from build123d import *

# Parameters (mm, degrees)
SKETCH1_R               = 18
SKETCH1_R_2             = 35
BOSS_EXTRUDE1_DEPTH     = 15
SKETCH1_3_R             = 35
SKETCH1_3_R_2           = 18
BOSS_EXTRUDE2_DEPTH     = 119
SKETCH1_4_R             = 18
SKETCH1_4_R_2           = 9
BOSS_EXTRUDE3_DEPTH     = 19
SKETCH1_5_W             = 56
SKETCH1_5_H             = 75
BOSS_EXTRUDE4_DEPTH     = 65
SKETCH2_R               = 14
CUT_EXTRUDE1_DEPTH      = 85.30367726
CUT_EXTRUDE1_DEPTH_BACK = 65
SKETCH3_R               = 24
SKETCH3_R_2             = 12.5
BOSS_EXTRUDE5_DEPTH     = 65
SKETCH1_6_R             = 18
CUT_EXTRUDE3_DEPTH      = 263
SKETCH3_3_R             = 12.5
CUT_EXTRUDE4_DEPTH      = 263


with BuildPart() as part:
    # Sketch1 → Boss-Extrude1 (new body)
    with BuildSketch(Plane(origin=(0, 0, 0), x_dir=(1, 0, 0), z_dir=(0, 1, 0))):
        with BuildLine():
            ThreePointArc((23.30367726, -61), (10.58036287, -81.76336426), (-13.696259751, -79.854013967))
            Line((-13.696259751, -79.854013967), (-72, -37.5))
            Line((-72, -37.5), (-72, 37.5))
            Line((-72, 37.5), (-15.87486298, 86.999686813))
            ThreePointArc((-15.87486298, 86.999686813), (9.874292088, 90.874605271), (24, 69))
            Line((24, 69), (24, 38.065732621))
            ThreePointArc((24, 38.065732621), (44.998138968, -0.409254655), (23.30367726, -38.495955971))
            Line((23.30367726, -38.495955971), (23.30367726, -61))
        make_face()
        with Locations((0, 69)):
            Circle(SKETCH1_R, mode=Mode.SUBTRACT)
        Circle(SKETCH1_R_2, mode=Mode.SUBTRACT)
        with Locations((0, -61)):
            Circle(SKETCH1_R, mode=Mode.SUBTRACT)
    extrude(amount=BOSS_EXTRUDE1_DEPTH)

    # Sketch1_3 → Boss-Extrude2 (add)
    with BuildSketch(Plane(origin=(0, 0, 0), x_dir=(1, 0, 0), z_dir=(0, 1, 0))):
        Circle(SKETCH1_3_R)
        Circle(SKETCH1_3_R_2, mode=Mode.SUBTRACT)
    extrude(amount=BOSS_EXTRUDE2_DEPTH)

    # Sketch1_4 → Boss-Extrude3 (add)
    with BuildSketch(Plane(origin=(0, 0, 0), x_dir=(1, 0, 0), z_dir=(0, 1, 0))):
        with Locations((0, -61)):
            Circle(SKETCH1_4_R)
        with Locations((0, -61)):
            Circle(SKETCH1_4_R_2, mode=Mode.SUBTRACT)
        with Locations((0, 69)):
            Circle(SKETCH1_4_R)
        with Locations((0, 69)):
            Circle(SKETCH1_4_R_2, mode=Mode.SUBTRACT)
    extrude(amount=BOSS_EXTRUDE3_DEPTH)

    # Sketch1_5 → Boss-Extrude4 (add)
    with BuildSketch(Plane(origin=(0, 0, 0), x_dir=(1, 0, 0), z_dir=(0, 1, 0))):
        with Locations((-100, 0)):
            Rectangle(SKETCH1_5_W, SKETCH1_5_H)
    extrude(amount=BOSS_EXTRUDE4_DEPTH)

    # Sketch2 → Cut-Extrude1 (cut, two sides)
    with BuildSketch(Plane.XY) as cut_extrude1_sk:
        with BuildLine():
            Line((-72, 65), (-100, 65))
            ThreePointArc((-100, 65), (-80.201010127, 56.798989873), (-72, 37))
            Line((-72, 37), (-72, 65))
        make_face()
        with BuildLine():
            Line((-128, 65), (-128, 37))
            ThreePointArc((-128, 37), (-119.798989873, 56.798989873), (-100, 65))
            Line((-100, 65), (-128, 65))
        make_face()
        with Locations((-100, 37)):
            Circle(SKETCH2_R)
    extrude(amount=CUT_EXTRUDE1_DEPTH, mode=Mode.SUBTRACT)
    extrude(cut_extrude1_sk.sketch, amount=-CUT_EXTRUDE1_DEPTH_BACK, mode=Mode.SUBTRACT)

    # Sketch3 → Boss-Extrude5 (add)
    with BuildSketch(Plane(origin=(0, 0, 0), x_dir=(0, 0, -1), z_dir=(1, 0, 0))):
        with Locations((0, 89)):
            Circle(SKETCH3_R)
        with Locations((0, 89)):
            Circle(SKETCH3_R_2, mode=Mode.SUBTRACT)
    extrude(amount=BOSS_EXTRUDE5_DEPTH)

    # Sketch1_6 → Cut-Extrude3 (cut)
    with BuildSketch(Plane(origin=(0, 0, 0), x_dir=(1, 0, 0), z_dir=(0, 1, 0))):
        Circle(SKETCH1_6_R)
    extrude(amount=CUT_EXTRUDE3_DEPTH, mode=Mode.SUBTRACT)

    # Sketch3_3 → Cut-Extrude4 (cut)
    with BuildSketch(Plane(origin=(0, 0, 0), x_dir=(0, 0, -1), z_dir=(1, 0, 0))):
        with Locations((0, 89)):
            Circle(SKETCH3_3_R)
    extrude(amount=CUT_EXTRUDE4_DEPTH, mode=Mode.SUBTRACT)


solid = part.part
CAD build for the part. Positions are in the model's coordinates, mm. A direction names the side the tool comes from. Coordinates: 2 decimals unless noted, no trailing zeros. Write each loop counter-clockwise with the first axis right and the second up, starting at its lowest first coordinate (ties: lowest second). Pieces come first, ordered by that corner, then holes. Notation, with made-up numbers: (50.25, 58) - (67.25, 58) arc R8 ccw to (67.25, 64) - close; hole circle Ø1 at (88.25, -19). An arc over 180 degrees is marked (long way). Use a Markdown table: item, result. Add a question column.
Item 1: Band-saw the part on C-C, the plane y = 10.5. Give the cut face in (x, z).
Item 2: 3-axis set-ups, long thin cutter, end or side, ignore diameter. For faces 1 (the face through (23.304, 7, 50)), 2 (the face through (-8.3, 19, 56.7)), 3 (the face through (-2.343, 16.972, -86.847)): which of +Z, -Z, +X, -X, +Y, -Y reach the whole face in a straight line?
Item 3: Flat gauge pins, fed straight in: pin 1 (17 mm diameter, centred on x = -102, y = 17, fed in from -Z); pin 2 (7.5 mm diameter, centred on y = 7.5, z = 47, fed in from +X); pin 3 (4.5 mm diameter, centred on y = 9, z = -48.5, fed in from +X). Where does each tip first touch, or does it go through?
Item 4: Band-saw the part on B-B, the plane x = -100. Give the cut face in (y, z), and give its area (4 significant figures).
Item 5: Band-saw the part on D-D, the plane x = 0. Give the cut face in (y, z).
Item 6: Mould opens along Y. For faces 4 (the face through (-34.966, 66.272, -1.539)), 5 (the face through (49.35, 79.81, -22.17)), 6 (the face through (-100, 18, 37.5)), 7 (the face through (-8.3, 19, -73.3)) say: pulls with the +Y half, pulls with the -Y half, needs draft (parallel to the pull), parting line crosses it, or undercut.
Item 7: Drill centre lines: L1, parallel to Z at x = 27.75, y = 89; L2, parallel to Y at x = 26.5, z = 0; L3, parallel to Z at x = -15, y = 81. Where is each one in solid material? Low to high. Write a range as from..to.
Item 8: Band-saw the part on A-A, the plane z = 0. Give the cut face in (x, y), and give its area (3 significant figures).
Numbers:
| question | item | result |
|---|---|---|
| 1 | outline | (-128, -37.5) - (-72, -37.5) - (-15.87, -87) arc R24 ccw to (24, -69) - (24, -38.07) arc R45 ccw to (23.3, 38.5) - (23.3, 61) arc R23.3 ccw to (-13.7, 79.85) - (-72, 37.5) - (-128, 37.5) - close; hole circle Ø36 at (0, 0); hole circle Ø18 at (0, -69); hole circle Ø18 at (0, 61) |
| 2 | face 1 | +Z, +X, +Y, -Y |
| 2 | face 2 | +Z, +X, -X, +Y |
| 2 | face 3 | +Y |
| 3 | pin 1 | z = -37.5 |
| 3 | pin 2 | x = 23.3 |
| 3 | pin 3 | x = 24 |
| 4 | outline | (0, -37.5) - (23, -37.5) - (23, 37.5) - (0, 37.5) - close; (51, -37.5) - (65, -37.5) - (65, 37.5) - (51, 37.5) - close |
| 4 | area | 2,775 mm2 |
| 5 | outline | (0, -93) - (15, -93) - (15, -87) - (19, -87) - (19, -78) - (0, -78) - close; (0, -60) - (19, -60) - (19, -51) - (15, -51) - (15, -35) - (119, -35) - (119, -18) - (0, -18) - close; (0, 18) - (119, 18) - (119, 35) - (15, 35) - (15, 43) - (19, 43) - (19, 52) - (0, 52) - close; (0, 70) - (19, 70) - (19, 79) - (15, 79) - (15, 84.3) - (0, 84.3) - close |
| 6 | face 4 | undercut |
| 6 | face 5 | undercut |
| 6 | face 6 | needs draft |
| 6 | face 7 | pulls with the +Y half |
| 7 | L1 | -24..-12.5, 12.5..24 |
| 7 | L2 | 0..76.5, 101.5..119 |
| 7 | L3 | -31.62..-9.95, 9.95..31.62 |
| 8 | outline | (-128, 0) - (-18, 0) - (-18, 119) - (-35, 119) - (-35, 15) - (-72, 15) - (-72, 37) arc R28 ccw to (-128, 37) - close; (18, 0) - (45, 0) - (45, 15) - (35, 15) - (35, 65) - (65, 65) - (65, 76.5) - (18, 76.5) - close; (18, 101.5) - (65, 101.5) - (65, 113) - (35, 113) - (35, 119) - (18, 119) - close; hole circle Ø28 at (-100, 37) |
| 8 | area | 7,700 mm2 |
